Autodesk Inventor part; units mm, degrees
ref_plane "Work Plane2" through (0, -15.1765, 0) normal (0, 1, 0) x (-1, 0, 0)
ref_plane "YZ Plane" through (0, 0, 0) normal (1, 0, 0) x (0, 1, 0)
ref_plane "XY Plane" through (0, 0, 0) normal (0, 0, 1) x (1, 0, 0)
sketch "Sketch1" plane through (0, 0, 0) normal (0, 0, 1) x (1, 0, 0)
  circle A0 centre (0, 0) radius 38.1
  dimension "d0" = 76.2
extrude "Extrusion1" add sketch "Sketch1" against normal blind 9.525
sketch "Sketch2" plane through (0, 0, -9.525) normal (0, 0, -1) x (-1, 0, 0)
  circle A0 centre (0, 0) radius 15.1765
  dimension "d3" = 30.353
extrude "Extrusion2" add sketch "Sketch2" along normal blind 15.875
sketch "Sketch3" plane through (0, 0, 0) normal (0, 0, 1) x (1, 0, 0)
  arc A0 (-1.1906, 4.8732) -> (1.1906, 4.8732) centre (0, 0) ccw
  line L0 (-1.1906, 4.8732) -> (-1.1906, 3.4285)
  line L1 (-1.1906, 3.4285) -> (1.1906, 3.4285)
  line L2 (1.1906, 3.4285) -> (1.1906, 4.8732)
  circle A1 centre (0, 0) radius 15.1765
  dimension "d6" = 10.033
  dimension "d7" = 2.3813
  dimension "d8" = 1.4446
  dimension "d15" = 10.16
extrude "Extrusion3" cut sketch "Sketch3" against normal through all contours L0 L1 L2 A0
ref_plane "Work Plane2" through (0, -15.1765, 0) normal (0, 1, 0) x (-1, 0, 0)
sketch "Sketch4" plane through (0, -15.1765, 0) normal (0, 1, 0) x (-1, 0, 0)
  line L0 (-15.1765, -9.525) -> (-15.1765, -25.4)
  line L1 (15.1765, -9.525) -> (15.1765, -25.4)
  line L2 (-38.1, -9.525) -> (38.1, -9.525)
  line L3 (-15.1765, -25.4) -> (15.1765, -25.4)
  line L4 (0, -25.4) -> (0, -9.525) construction
  point P0 (0, 0)
  point P1 (0, -17.4625)
hole "Hole1" at (0, -15.1765, -17.4625) direction (0, 1, 0) diameter 5.1054 depth 11.43 counterbore diameter 6.5278 counterbore depth 7.874
sketch "Sketch5" plane through (0, 0, -9.525) normal (0, 0, -1) x (-1, 0, 0)
  circle A0 centre (0, 0) radius 25.4 construction
  line L0 (-28.0674, 5.9618) -> (-22.0201, 3.0404)
  line L1 (-22.0201, 3.0404) -> (-22.1276, 2.1359)
  line L2 (-22.1276, 2.1359) -> (-28.6914, 0.7139)
  line L3 (-28.6914, 0.7139) -> (-28.5844, 1.6133)
  line L4 (-28.5844, 1.6133) -> (-23.139, 2.7381)
  line L5 (-23.139, 2.7381) -> (-28.1689, 5.1084)
  line L6 (-28.1689, 5.1084) -> (-28.0674, 5.9618)
  spline S0 degree 2 poles (-23.232, 10.4675) (-21.6233, 9.8922) (-20.4509, 8.4181) (-20.7992, 7.4442) knots 0 0 0 1 2 2 2
  spline S1 degree 2 poles (-20.7992, 7.4442) (-21.1527, 6.4557) (-23.0196, 6.0796) (-24.5944, 6.6428) knots 0 0 0 1 2 2 2
  spline S2 degree 2 poles (-24.5944, 6.6428) (-26.2127, 7.2216) (-27.3754, 8.6922) (-27.0254, 9.6709) knots 0 0 0 1 2 2 2
  spline S3 degree 2 poles (-27.0254, 9.6709) (-26.6736, 10.6545) (-24.7921, 11.0255) (-23.232, 10.4675) knots 0 0 0 1 2 2 2
  spline S4 degree 2 poles (-21.7775, 8.7887) (-22.0315, 9.0107) (-22.9077, 9.4334) (-23.5231, 9.6535) knots 0 0 0 1 2 2 2
  spline S5 degree 2 poles (-23.5231, 9.6535) (-24.1384, 9.8735) (-25.0792, 10.1007) (-25.4277, 10.0887) knots 0 0 0 1 2 2 2
  spline S6 degree 2 poles (-25.4277, 10.0887) (-25.7763, 10.0768) (-26.242, 9.7679) (-26.3616, 9.4335) knots 0 0 0 1 2 2 2
  spline S7 degree 2 poles (-26.3616, 9.4335) (-26.4812, 9.0992) (-26.3204, 8.5553) (-26.0506, 8.3167) knots 0 0 0 1 2 2 2
  spline S8 degree 2 poles (-26.0506, 8.3167) (-25.7886, 8.0864) (-24.8895, 7.6665) (-24.3032, 7.4568) knots 0 0 0 1 2 2 2
  spline S9 degree 2 poles (-24.3032, 7.4568) (-23.6733, 7.2315) (-22.8025, 7.0075) (-22.428, 7.0157) knots 0 0 0 1 2 2 2
  spline S10 degree 2 poles (-22.428, 7.0157) (-22.0763, 7.0211) (-21.5878, 7.3327) (-21.463, 7.6816) knots 0 0 0 1 2 2 2
  spline S11 degree 2 poles (-21.463, 7.6816) (-21.3451, 8.0111) (-21.5059, 8.5549) (-21.7775, 8.7887) knots 0 0 0 1 2 2 2
  spline S12 degree 2 poles (-23.8527, 14.6142) (-23.9751, 14.4177) (-24.1212, 13.9691) (-24.1639, 13.735) knots 0 0 0 1 2 2 2
  spline S13 degree 2 poles (-24.1639, 13.735) (-24.1985, 13.5141) (-24.2017, 13.1584) (-24.1944, 13.0144) knots 0 0 0 1 2 2 2
  line L7 (-24.1944, 13.0144) -> (-24.2216, 12.9707)
  line L8 (-24.2216, 12.9707) -> (-24.986, 13.4468)
  spline S14 degree 2 poles (-24.986, 13.4468) (-24.9658, 13.7616) (-24.6677, 14.6975) (-24.4419, 15.0601) knots 0 0 0 1 2 2 2
  spline S15 degree 2 poles (-24.4419, 15.0601) (-24.2134, 15.427) (-23.7248, 15.8805) (-23.4288, 16.0053) knots 0 0 0 1 2 2 2
  spline S16 degree 2 poles (-23.4288, 16.0053) (-23.1116, 16.135) (-22.4657, 16.0722) (-22.1337, 15.8655) knots 0 0 0 1 2 2 2
  spline S17 degree 2 poles (-22.1337, 15.8655) (-21.6882, 15.588) (-21.3801, 14.5837) (-21.5485, 14.1187) knots 0 0 0 1 2 2 2
  line L9 (-21.5485, 14.1187) -> (-21.496, 14.0861)
  spline S18 degree 2 poles (-21.496, 14.0861) (-21.355, 14.2346) (-20.9556, 14.5254) (-20.695, 14.5935) knots 0 0 0 1 2 2 2
  spline S19 degree 2 poles (-20.695, 14.5935) (-20.4387, 14.6642) (-19.8189, 14.5692) (-19.4651, 14.3488) knots 0 0 0 1 2 2 2
  spline S20 degree 2 poles (-19.4651, 14.3488) (-19.1026, 14.123) (-18.6418, 13.4905) (-18.5474, 13.1164) knots 0 0 0 1 2 2 2
  spline S21 degree 2 poles (-18.5474, 13.1164) (-18.4497, 12.7282) (-18.6126, 11.9021) (-18.8765, 11.4784) knots 0 0 0 1 2 2 2
  spline S22 degree 2 poles (-18.8765, 11.4784) (-19.1295, 11.0722) (-19.8212, 10.3997) (-20.1253, 10.2132) knots 0 0 0 1 2 2 2
  line L10 (-20.1253, 10.2132) -> (-20.8897, 10.6893)
  line L11 (-20.8897, 10.6893) -> (-20.857, 10.7417)
  spline S23 degree 2 poles (-20.857, 10.7417) (-20.5496, 10.8655) (-19.765, 11.4438) (-19.5283, 11.8238) knots 0 0 0 1 2 2 2
  spline S24 degree 2 poles (-19.5283, 11.8238) (-19.3896, 12.0466) (-19.2519, 12.5791) (-19.321, 12.8283) knots 0 0 0 1 2 2 2
  spline S25 degree 2 poles (-19.321, 12.8283) (-19.3928, 13.0731) (-19.682, 13.4654) (-19.9746, 13.6477) knots 0 0 0 1 2 2 2
  spline S26 degree 2 poles (-19.9746, 13.6477) (-20.2673, 13.83) (-20.7534, 13.8963) (-20.9578, 13.8114) knots 0 0 0 1 2 2 2
  spline S27 degree 2 poles (-20.9578, 13.8114) (-21.1622, 13.7266) (-21.5036, 13.3633) (-21.656, 13.1187) knots 0 0 0 1 2 2 2
  line L12 (-21.656, 13.1187) -> (-21.8464, 12.813)
  line L13 (-21.8464, 12.813) -> (-22.4448, 13.1857)
  line L14 (-22.4448, 13.1857) -> (-22.2952, 13.4259)
  spline S28 degree 2 poles (-22.2952, 13.4259) (-21.9932, 13.9107) (-22.0753, 14.8106) (-22.5165, 15.0854) knots 0 0 0 1 2 2 2
  spline S29 degree 2 poles (-22.5165, 15.0854) (-22.7218, 15.2133) (-23.1124, 15.2383) (-23.2786, 15.166) knots 0 0 0 1 2 2 2
  spline S30 degree 2 poles (-23.2786, 15.166) (-23.4547, 15.0878) (-23.7357, 14.8021) (-23.8527, 14.6142) knots 0 0 0 1 2 2 2
  dimension "d24" = 50.8
extrude "Extrusion4" cut sketch "Sketch5" against normal blind 2.54
equation "\"d0\" = outerDiameter"
equation "\"d1\" = handleThickness"
equation "\"d3\" = shaftOutsideDiameter"
equation "\"d4\" = shaftLength"
equation "\"d6\" = shaftDiameter"
equation "\"d7\" = keyWidth"
equation "\"d8\" = keyDepth"
equation "\"outerDiameter\" = 76.2"
equation "\"handleThickness\" = 9.525"
equation "\"totalLength\" = 25.4"
equation "\"shaftDiameter\" = 10.033"
equation "\"keyWidth\" = 2.38125"
equation "\"keyDepth\" = 1.44462"
equation "\"shaftLength\" = totalLength - handleThickness"
equation "\"shaftOutsideDiameter\" = shaftDiameter + 2 * setScrewDepth"
equation "\"setScrewDepth\" = 10.16"
equation "\"setScrewWorkPlane\" = 0.5 * shaftOutsideDiameter"
equation "\"d16\" = -setScrewWorkPlane"
properties part number "celestronMountDecHandle" material "PC/ABS Plastic"
Model file for the job. Use its own axes, mm. A direction names the side the tool comes from. Give positions to 0.01 mm unless a question says otherwise; leave off trailing zeros. Loops run counter-clockwise (first coordinate to the right, second up) from the corner with the lowest first, then second, coordinate; pieces in that order, holes last. Notation, with made-up numbers: (4.25, 15) - (57.25, 15) arc R28 cw to (57.25, 48) - close; hole circle Ø7 at (-20, 36). An arc over 180 degrees is marked (long way). Use one line per item in the form item = value.
(1) Pull direction Z, two halves, no side cores. Call faces 1 (the face through (24, 7, -6.985)), 2 (the face through (25.6, 3.9, -8.3)), 3 (the face through (3, -7.302, -17)): pulls with the +Z half, pulls with the -Z half, needs draft (parallel to the pull), parting line crosses it, or undercut.
Determined:
face_1 = pulls with the -Z half
face_2 = needs draft
face_3 = undercut
(2) Cut at D-D (z = -23.25). Give the cut face in (x, y).
Determined:
outline = circle Ø30.35 at (0, 0); hole (-1.19, 3.43) - (-1.19, 4.87) arc R5.02 ccw (long way) to (1.19, 4.87) - (1.19, 3.43) - close
(3) Cut at A-A (x = 0). Give the cut face in (y, z) (1 decimal), then the cut area to 3 significant figures.
Determined:
outline = (-38.1, -9.5) - (-15.2, -9.5) - (-15.2, -14.2) - (-7.3, -14.2) - (-7.3, -14.9) - (-5, -14.9) - (-5, 0) - (-38.1, 0) - close; (-15.2, -25.4) - (-5, -25.4) - (-5, -20) - (-7.3, -20) - (-7.3, -20.7) - (-15.2, -20.7) - close; (3.4, -25.4) - (15.2, -25.4) - (15.2, -9.5) - (38.1, -9.5) - (38.1, 0) - (3.4, 0) - close
area = 930 mm^2
(4) Cut at B-B (z = -2.75). Give the cut face in (x, y).
Determined:
outline = circle Ø76.2 at (0, 0); hole (-1.19, 3.43) - (-1.19, 4.87) arc R5.02 ccw (long way) to (1.19, 4.87) - (1.19, 3.43) - close
(5) 3-axis set-ups, long thin cutter, end or side, ignore diameter. For faces 4 (the face through (24, 9, -9.525)), 5 (the face through (-0.112, -6.121, -14.912)), 6 (the face through (0, 3.428, -13)), 7 (the face through (25.9, 2.168, -8.273)): which of +Z, -Z, +X, -X, +Y, -Y reach the whole face in a straight line?
Determined:
face_4 = -Z, +X, +Y, -Y
face_5 = -Y
face_6 = +Z, -Z
face_7 = -Z
(6) Drill centre lines: L1, parallel to Z at x = -18, y = 6 (3 decimals); L2, parallel to Z at x = 0, y = -9.75; L3, parallel to Y at x = 1.5, z = -14.5. Where is each one in solid material? Low to high.
Determined:
L1 = -9.525 to 0
L2 = -25.4 to -20.73, -14.2 to 0
L3 = -15.1 to -4.79, 4.79 to 15.1
(7) Drop flat-ended pins along their axis: P1, Ø4.5, axis at x = 22.5, y = 14, coming from the -Z side (3 decimals); P2, Ø1.6, axis at y = 4, z = -11, coming from the +X side; P3, Ø6, axis at y = -11, z = -3.5, coming from the +X side; P4, Ø6, axis at x = 0, y = 0, coming from the +Z side. Give the stop position or say it passes through.
Determined:
P1 = -9.525
P2 = 14.84
P3 = 37.25
P4 = through
(8) Cut at C-C (y = -9.5). Give the cut face in (x, z) (1 decimal).
Determined:
outline = (-36.9, -9.5) - (-11.8, -9.5) - (-11.8, -25.4) - (11.8, -25.4) - (11.8, -9.5) - (36.9, -9.5) - (36.9, 0) - (-36.9, 0) - close; hole circle Ø6.5 at (0, -17.5)
